Autodesk Inventor part; units mm, degrees
ref_plane "YZ Plane" through (0, 0, 0) normal (1, 0, 0) x (0, 1, 0)
ref_plane "XZ Plane" through (0, 0, 0) normal (0, 1, 0) x (-1, 0, 0)
ref_plane "XY Plane" through (0, 0, 0) normal (0, 0, 1) x (1, 0, 0)
sketch "草图2" plane through (0, 0, 0) normal (0, 1, 0) x (-1, 0, 0)
  line L0 (5, 0) -> (-5, 0) construction
  line L1 (5, 2.5) -> (-5, 2.5)
  line L2 (-5, -2.5) -> (5, -2.5)
  arc A0 (5, -2.5) -> (5, 2.5) centre (5, 0) ccw
  arc A1 (-5, 2.5) -> (-5, -2.5) centre (-5, 0) ccw
  line L3 (5, 0) -> (15, 0) construction
  circle A2 centre (5, 0) radius 2
  circle A3 centre (-5, 0) radius 2
  point P0 (0, 0)
  point P1 (0, 0)
  dimension "d6" = 10
  dimension "d7" = 180
  dimension "d8" = 5
  dimension "d9" = 4
  dimension "d10" = 4
extrude "拉伸1" add sketch "草图2" along normal blind 5
sketch "草图3" plane through (0, 5, 0) normal (0, 1, 0) x (1, 0, 0)
  line L0 (5, 0) -> (75.7107, 70.7107) construction
  line L1 (6.7678, -1.7678) -> (77.4784, 68.9429)
  line L2 (73.9429, 72.4784) -> (3.2322, 1.7678)
  arc A0 (3.2322, 1.7678) -> (6.7678, -1.7678) centre (5, 0) ccw
  arc A1 (77.4784, 68.9429) -> (73.9429, 72.4784) centre (75.7107, 70.7107) ccw
  line L3 (5, 0) -> (105, 0) construction
  line L4 (5, 0) -> (75.7107, -70.7107) construction
  line L5 (3.2322, -1.7678) -> (73.9429, -72.4784)
  line L6 (77.4784, -68.9429) -> (6.7678, 1.7678)
  arc A2 (6.7678, 1.7678) -> (3.2322, -1.7678) centre (5, 0) ccw
  arc A3 (73.9429, -72.4784) -> (77.4784, -68.9429) centre (75.7107, -70.7107) ccw
  line L7 (5, 0) -> (105, 0) construction
  point P0 (0, 0)
  point P1 (40.3553, 35.3553)
  point P2 (40.3553, -35.3553)
  dimension "d13" = 100
  dimension "d14" = 45
  dimension "d15" = 5
  dimension "d16" = 100
  dimension "d17" = 45
  dimension "d18" = 5
extrude "拉伸2" add sketch "草图3" against normal blind 5
sketch "草图4" plane through (0, 5, 0) normal (0, 1, 0) x (1, 0, 0)
  circle A0 centre (5, 0) radius 2
  point P0 (0, 0)
  dimension "d21" = 4
extrude "拉伸3" cut sketch "草图4" against normal through all
fillet "圆角1" radius 2 4 edges at (3, 0, 0) (3, 5, 0) (-3, 5, 0) (-3, 0, 0)
properties part number "压缩杆"
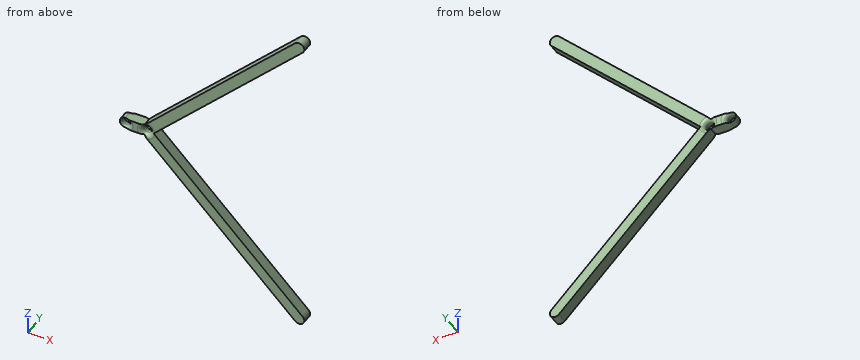
Check sheet for the modelled part. Datum: model origin and axes. Units: mm. Round coordinates to 2 decimals unless told otherwise and drop trailing zeros. Order: outer loops, then holes, each group sorted by start corner. A loop starts at its lowest first (then second) coordinate and runs counter-clockwise, first axis right, second up.
(1) Scan lines: probe 1 along Z at (x, y) = (-5, 2.3); probe 2 along Z at (x, y) = (12.5, 3.85); probe 3 along X at (y, z) = (1.3, 1). Record each from-to range of solid material in increasing order.
(2) Go/stop test with flat-tipped pins: P1, Ø1.5, axis at x = 0.5, y = 2.5, coming from the +Z side; P2, Ø3, axis at x = 18.5, y = 3, coming from the -Z side. Record where each tip stops, or that it passes through.
(3) Cross-section at C-C, the plane z = 52.5. Enter the section's corners in (x, y), and give its area (3 significant figures).
(4) Cross-section at A-A, the plane x = 17.5. Enter the section's corners in (y, z).
(5) Cross-section at D-D, the plane z = 20. Enter the section's corners in (x, y), and give its area (3 significant figures).
(6) Cross-section at B-B, the plane x = 70. Enter the section's corners in (y, z).
Check sheet entries:
1. probe 1: z = -2.5 to -2, 2 to 2.5
1. probe 2: z = -11.04 to -3.96, 3.96 to 11.04
1. probe 3: x = -7.29 to -6.88, -3.12 to 3.12, 6.88 to 9.54
2. P1: stops at z = 2.5
2. P2: stops at z = -18.54
3. outline: (53.96, 0) - (61.04, 0) - (61.04, 5) - (53.96, 5) - close
3. area: 35.4 mm2
4. outline: (0, -16.04) - (5, -16.04) - (5, -8.96) - (0, -8.96) - close; (0, 8.96) - (5, 8.96) - (5, 16.04) - (0, 16.04) - close
5. outline: (21.46, 0) - (28.54, 0) - (28.54, 5) - (21.46, 5) - close
5. area: 35.4 mm2
6. outline: (0, -68.54) - (5, -68.54) - (5, -61.46) - (0, -61.46) - close; (0, 61.46) - (5, 61.46) - (5, 68.54) - (0, 68.54) - close
